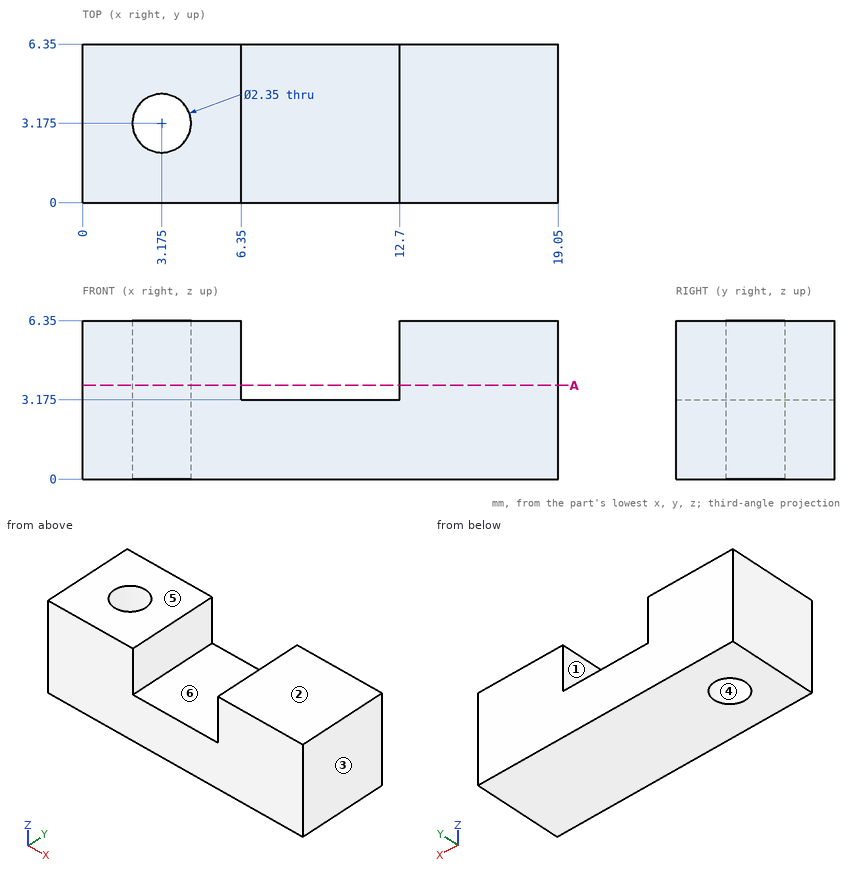
Verification items for this drawing (mm, ordinates from the low corner). A direction names the side the tool comes from. Coordinates: 2 decimals unless noted, no trailing zeros. Answer in a Markdown table with one row per item. Add a question column.
1. Draft check along X on the marked faces 3, 4, 5 and 6. Enter one of: +X half, -X half, draft (parallel to the pull), parting line (faces both ways), or undercut.
2. Depth check by flat-ended pin: P1, Ø1.9, axis at x = 10, y = 2, coming from the +Z side (3 decimals); P2, Ø2, axis at x = 3.175, y = 3.175, coming from the -Z side. Enter the tip coordinate at first touch or a pass-through.
3. Material ranges on probe 1 along X at (y, z) = (5.75, 5.5); probe 2 along X at (y, z) = (2.5, 3.5); probe 3 along X at (y, z) = (2.75, 5.5), recorded low to high. Write a range as [from, to].
4. Access from +Z, -Z, +X, -X, +Y, -Y to the whole of each face (thin tool, end or side, straight path). Record for the marked faces 1 and 2.
5. Section check A-A, the plane z = 3.75. Give the number of separate pieces and of enclosed holes in the cut face, then the cut area to 3 significant figures.
Derived:
| question | item | result |
|---|---|---|
| 1 | face 3 | +X half |
| 1 | face 4 | undercut |
| 1 | face 5 | draft |
| 1 | face 6 | undercut |
| 2 | P1 | stops at z = 3.175 |
| 2 | P2 | passes through |
| 3 | probe 1 | x = [0, 6.35], [12.7, 19.05] |
| 3 | probe 2 | x = [0, 2.21], [4.14, 6.35], [12.7, 19.05] |
| 3 | probe 3 | x = [0, 2.08], [4.27, 6.35], [12.7, 19.05] |
| 4 | face 1 | +Z, +Y, -Y |
| 4 | face 2 | +Z, +X, -X, +Y, -Y |
| 5 | separate pieces | 2 |
| 5 | enclosed holes | 1 |
| 5 | area | 76.3 mm² |
